Model file for the job. Use its own axes, mm. A direction names the side the tool comes from. Round coordinates to 2 decimals unless told otherwise and drop trailing zeros. Loops run counter-clockwise (first coordinate to the right, second up) from the corner with the lowest first, then second, coordinate; pieces in that order, holes last. Notation, with made-up numbers: (9.5, -6) - (55.5, -6) arc R17 cw to (55.5, 11) - close; hole circle Ø2 at (-19.5, 25). An arc over 180 degrees is marked (long way). Answer as a JSON object with one key per item and string values.
from build123d import *

# Parameters (mm, degrees)
F0_R            = 14
F1_DEPTH        = 8
F3_D            = 6
F4_D            = 2.4
F4_COPIES_COUNT = 3
F6_D            = 2.4
F6_DEPTH        = 14.001


# Not quite as in the source:
# - a pattern or mirror of a feature is missing from the dataset's text; its kind, count and spacing are read off the source's solid


with BuildPart() as f1:
    # F0 (on Top) → F1 (new body)
    with BuildSketch(Plane.XY):
        Circle(F0_R)
    extrude(amount=F1_DEPTH)

    # F3 (through all)
    with Locations(Plane.XY.offset(8)):
        with Locations((0, 0)):
            Hole(F3_D / 2)

    # F4 (through all)
    with Locations(Plane.XY.offset(8)):
        with Locations((-10.5, 0)):
            f4 = Hole(F4_D / 2)

    # F4_copies: F4 ×3 about axis
    f4_copies_axis = Axis((0, 0, 0), (0, 0, 1))
    for i in range(1, F4_COPIES_COUNT):
        add(f4.rotate(f4_copies_axis, i * 360 / F4_COPIES_COUNT), mode=Mode.SUBTRACT)

    # F6 (through all, one way)
    with BuildSketch(Plane(origin=(0, 0, 0), x_dir=(0, 1, 0), z_dir=(-1, 0, 0))):
        with Locations((0, -4)):
            Circle(F6_D / 2)
    extrude(amount=-F6_DEPTH, mode=Mode.SUBTRACT)


solid = f1.part
1) Slice it at D-D on z = 3.5. List the corners of the cut face in (x, y).
Values follow:
{"outline": "(2.79, -1.09) arc R3 cw (long way) to (2.79, 1.09) - (13.96, 1.09) arc R14 ccw (long way) to (13.96, -1.09) - close; hole circle Ø2.4 at (-10.5, 0); hole circle Ø2.4 at (5.25, -9.09); hole circle Ø2.4 at (5.25, 9.09)"}
2) Slice it at B-B on y = 0. List the corners of the cut face in (x, z).
Values follow:
{"outline": "(-14, 0) - (-11.7, 0) - (-11.7, 8) - (-14, 8) - close; (-9.3, 0) - (-3, 0) - (-3, 8) - (-9.3, 8) - close; (3, 0) - (14, 0) - (14, 2.8) - (3, 2.8) - close; (3, 5.2) - (14, 5.2) - (14, 8) - (3, 8) - close"}
3) Tool access for faces 1 (the cylindrical face through (-2.86, 0.9, 3.94)), 2 (the cylindrical face through (8.3, 0.65, 2.99)): list every direction of +Z, -Z, +X, -X, +Y, -Y with a clear straight run to the whole face (end or side of a thin tool).
Values follow:
{"face 1": "+Z, -Z", "face 2": "+X"}
4) Probe probe 1 along Z at (x, y) = (8, 0); probe 2 along Y at (x, z) = (0, 4); probe 3 along Y at (x, z) = (5.25, 6.25). List the from-to ranges inside material, lowest first.
Values follow:
{"probe 1": "0 to 2.8, 5.2 to 8", "probe 2": "-14 to -3, 3 to 14", "probe 3": "-12.98 to -10.29, -7.89 to 7.89, 10.29 to 12.98"}
5) Slice it at C-C on y = -9. List the corners of the cut face in (x, z), then the cut area to 3 significant figures.
Values follow:
{"outline": "(-10.72, 0) - (4.05, 0) - (4.05, 8) - (-10.72, 8) - close; (6.45, 0) - (10.72, 0) - (10.72, 8) - (6.45, 8) - close", "area": "152 mm²"}
6) Two-plate mould, pull along X, no slides. Class faces 3 (the cylindrical face through (12.932, -5.362, 3.944)), 4 (the cylindrical face through (6.202, -9.823, 3.944)), 5 (the flat face through (-3.3, 0.2, 8)): pulls with the +X half, pulls with the -X half, needs draft (parallel to the pull), parting line crosses it, or undercut.
Values follow:
{"face 3": "parting line crosses it", "face 4": "undercut", "face 5": "needs draft"}
7) Slice it at A-A on x = 0. List the corners of the cut face in (y, z), then the cut area to 3 significant figures.
Values follow:
{"outline": "(-14, 0) - (-3, 0) - (-3, 8) - (-14, 8) - close; (3, 0) - (14, 0) - (14, 8) - (3, 8) - close", "area": "176 mm²"}
8) Drop flat-ended pins along their axis: P1, Ø2, axis at y = -2.5, z = 3, coming from the -X side; P2, Ø1, axis at x = -10, z = 3, coming from the +Y side. Give the stop position or say it passes through.
Values follow:
{"P1": "x = -13.92", "P2": "y = 10.28"}
